Design review of the part built by this model. Coordinates are the model's own, in mm. A direction names the side the tool comes from. Coordinates: 2 decimals unless noted, no trailing zeros. Write each loop counter-clockwise with the first axis right and the second up, starting at its lowest first coordinate (ties: lowest second). Pieces come first, ordered by that corner, then holes. Notation, with made-up numbers: (43.5, 89) - (77.5, 89) arc R14 cw to (77.5, 103) - close; hole circle Ø6 at (-37.75, 48.5). An arc over 180 degrees is marked (long way). Answer as a JSON object with one key per item and string values.
```python
from build123d import *

# Parameters (mm, degrees)
F1_DEPTH  = 27.94
F2_R      = 2.032
F3_DEPTH  = 2.54
F4_R      = 2.032
F5_DEPTH  = 2.54
F6_SIZE   = 2.54
F7_W      = 27.94
F7_H      = 1.27
F8_DEPTH  = 1.27
F9_W      = 27.94
F9_H      = 1.27
F10_DEPTH = 1.27


with BuildPart() as f1:
    # F0 (on Right) → F1 (new body)
    with BuildSketch(Plane.YZ):
        Polygon((0, 30.226001516), (-35.56, 30.226001516), (-35.56, 27.686001516), (-2.54, 27.686001516), (-2.54, -0.253998484), (-35.56, -0.253998484), (-35.56, -2.793998484), (0, -2.793998484), align=None)
    extrude(amount=F1_DEPTH)

    # F2 (on face) → F3 (cut, through all)
    with BuildSketch(Plane.XY.offset(30.226001516)):
        with Locations((9.144, -10.16)):
            Circle(F2_R)
        with Locations((19.3227036137, -27.7468244076)):
            Circle(F2_R)
        with BuildLine():
            Line((21.8533518069, -16.9894844152), (6.6133518069, -16.9894844152))
            ThreePointArc((6.6133518069, -16.9894844152), (4.6494240183, -18.9534122038), (6.6133518069, -20.9173399924))
            Line((6.6133518069, -20.9173399924), (21.8533518069, -20.9173399924))
            ThreePointArc((21.8533518069, -20.9173399924), (23.8172795954, -18.9534122038), (21.8533518069, -16.9894844152))
        make_face()
        with BuildLine():
            ThreePointArc((21.8439999996, -14.605), (26.2890393498, -10.1786250789), (21.8814072278, -5.715))
            Line((21.8814072278, -5.715), (16.8014072278, -5.715))
            ThreePointArc((16.8014072278, -5.715), (12.3189606494, -10.1412175195), (16.7639999996, -14.605))
            Line((16.7639999996, -14.605), (21.8439999996, -14.605))
        make_face()
        with BuildLine():
            ThreePointArc((11.7027036137, -32.1918244076), (16.1477036137, -27.7468244076), (11.7027036137, -23.3018244076))
            Line((11.7027036137, -23.3018244076), (6.6227036137, -23.3018244076))
            ThreePointArc((6.6227036137, -23.3018244076), (2.1777036137, -27.7468244076), (6.6227036137, -32.1918244076))
            Line((6.6227036137, -32.1918244076), (11.7027036137, -32.1918244076))
        make_face()
    extrude(amount=-F3_DEPTH, mode=Mode.SUBTRACT)

    # F4 (on face) → F5 (cut, through all)
    with BuildSketch(Plane(origin=(0, 0, -2.793998484), x_dir=(1, 0, 0), z_dir=(0, 0, -1))):
        with Locations((9.1366654938, 27.746792541)):
            Circle(F4_R)
        with Locations((19.3154241667, 10.16)):
            Circle(F4_R)
        with BuildLine():
            Line((21.8460448303, 20.9173240591), (6.6060448303, 20.9173240591))
            ThreePointArc((6.6060448303, 20.9173240591), (4.6421170417, 18.9533962705), (6.6060448303, 16.9894684819))
            Line((6.6060448303, 16.9894684819), (21.8460448303, 16.9894684819))
            ThreePointArc((21.8460448303, 16.9894684819), (23.8099726188, 18.9533962705), (21.8460448303, 20.9173240591))
        make_face()
        with BuildLine():
            ThreePointArc((21.8356585741, 23.3013725448), (26.2811203019, 27.7276136907), (21.8741828399, 32.1922125373))
            Line((21.8741828399, 32.1922125373), (16.7951897592, 32.1922125373))
            ThreePointArc((16.7951897592, 32.1922125373), (12.3112037656, 27.7661383181), (16.7566654934, 23.3013725448))
            Line((16.7566654934, 23.3013725448), (21.8356585741, 23.3013725448))
        make_face()
        with BuildLine():
            ThreePointArc((11.6954241667, 5.715), (16.1404241667, 10.16), (11.6954241667, 14.605))
            Line((11.6954241667, 14.605), (6.6154241667, 14.605))
            ThreePointArc((6.6154241667, 14.605), (2.1704241667, 10.16), (6.6154241667, 5.715))
            Line((6.6154241667, 5.715), (11.6954241667, 5.715))
        make_face()
    extrude(amount=-F5_DEPTH, mode=Mode.SUBTRACT)

    # F6
    f6_edges = [f1.edges().sort_by_distance(p)[0] for p in [
        (13.97, -2.54, -0.253998),
        (13.97, -2.54, 27.686002),
    ]]
    chamfer(f6_edges, length=F6_SIZE)

    # F7 (on face) → F8 (join)
    with BuildSketch(Plane.XY.offset(-0.253998484)):
        with Locations((13.97, -34.925)):
            Rectangle(F7_W, F7_H)
    extrude(amount=F8_DEPTH)

    # F9 (on face) → F10 (join)
    with BuildSketch(Plane(origin=(0, 0, 27.686001516), x_dir=(1, 0, 0), z_dir=(0, 0, -1))):
        with Locations((13.97, 34.925)):
            Rectangle(F9_W, F9_H)
    extrude(amount=F10_DEPTH)


solid = f1.part
```
(1) For pin 1 (1 mm diameter, centred on x = 25, z = 11, fed in from -Y); pin 2 (6 mm diameter, centred on x = 15, z = 22.5, fed in from -Y); pin 3 (1 mm diameter, centred on x = 8, y = -28, fed in from +Z), all flat-tipped, find the tip position at first contact; note any pin that passes through.
Solved:
{"pin 1": "stops at y = -2.54", "pin 2": "stops at y = -2.89", "pin 3": "passes through"}
(2) Take a section at C-C, the plane x = 24.75. Write out the cut boundary in (y, z), and give its area (3 significant figures).
Solved:
{"outline": "(-35.56, -2.79) - (-31.1, -2.79) - (-31.1, -0.25) - (-34.29, -0.25) - (-34.29, 1.02) - (-35.56, 1.02) - close; (-35.56, 26.42) - (-34.29, 26.42) - (-34.29, 27.69) - (-13.52, 27.69) - (-13.52, 30.23) - (-35.56, 30.23) - close; (-24.39, -2.79) - (0, -2.79) - (0, 30.23) - (-6.8, 30.23) - (-6.8, 27.69) - (-5.08, 27.69) - (-2.54, 25.15) - (-2.54, 2.29) - (-5.08, -0.25) - (-24.39, -0.25) - close", "area": "227 mm^2"}
(3) Take a section at B-B, the plane y = -16.5. Write out the cut boundary in (x, z).
Solved:
{"outline": "(0, -2.79) - (27.94, -2.79) - (27.94, -0.25) - (0, -0.25) - close; (0, 27.69) - (27.94, 27.69) - (27.94, 30.23) - (0, 30.23) - close"}
(4) To check wall thickness, follow line 1 (X direction, y = -27, z = -1); line 2 (Z direction, x = 4.5, y = -34); line 3 (Y direction, x = 16.25, z = -0.5). State the ranges of each line that lie inside material, in increasing order. Write a range as from..to.
Solved:
{"line 1": "x = 0..7.25, 11.03..12.37, 26.22..27.94", "line 2": "z = -2.79..-0.25, 27.69..30.23", "line 3": "y = -35.56..-32.16, -23.33..-20.92, -16.99..0"}
(5) Tool access review of faces 4 (the face through (9, -23.302, 29)), 5 (the face through (26.28, -27.63, -1.54)), 6 (the face through (14, -34.29, 0)): name each direction out of +Z, -Z, +X, -X, +Y, -Y from which nothing blocks a thin tool from reaching the whole face with its end or side.
Solved:
{"face 4": "+Z", "face 5": "-Z", "face 6": "+X, -X"}
(6) The part is to be moulded in two halves that separate along Z. For faces 1 (the face through (14, -35, 26.416)), 2 (the face through (14, -22, -2.794)), 3 (the face through (27.94, -2, 15)), say which applies: pulls with the +Z half, pulls with the -Z half, needs draft (parallel to the pull), parting line crosses it, or undercut.
Solved:
{"face 1": "undercut", "face 2": "pulls with the -Z half", "face 3": "needs draft"}
(7) Take a section at A-A, the plane y = -10.16. Write out the cut boundary in (x, z), and give its area (3 significant figures).
Solved:
{"outline": "(0, -2.79) - (2.17, -2.79) - (2.17, -0.25) - (0, -0.25) - close; (0, 27.69) - (7.11, 27.69) - (7.11, 30.23) - (0, 30.23) - close; (11.18, 27.69) - (12.32, 27.69) - (12.32, 30.23) - (11.18, 30.23) - close; (16.14, -2.79) - (17.28, -2.79) - (17.28, -0.25) - (16.14, -0.25) - close; (21.35, -2.79) - (27.94, -2.79) - (27.94, -0.25) - (21.35, -0.25) - close; (26.29, 27.69) - (27.94, 27.69) - (27.94, 30.23) - (26.29, 30.23) - close", "area": "50.3 mm^2"}
(8) Take a section at D-D, the plane y = -31. Write out the cut boundary in (x, z).
Solved:
{"outline": "(0, -2.79) - (13.73, -2.79) - (13.73, -0.25) - (0, -0.25) - close; (0, 27.69) - (3.59, 27.69) - (3.59, 30.23) - (0, 30.23) - close; (14.73, 27.69) - (27.94, 27.69) - (27.94, 30.23) - (14.73, 30.23) - close; (24.87, -2.79) - (27.94, -2.79) - (27.94, -0.25) - (24.87, -0.25) - close"}
